The figure shows three views and two pictorial views of one solid part (mm, origin at its lowest corner). Answer the questions. Round coordinates to 2 decimals unless told otherwise and drop trailing zeros. Order: outer loops, then holes, each group sorted by start corner. A loop starts at its lowest first (then second) coordinate and runs counter-clockwise, first axis right, second up. Notation, with made-up numbers: (-26, 40) - (10, 40) arc R21 cw to (10, 60) - close; hole circle Ø8 at (-5.5, -5.5). An arc over 180 degrees is marked (long way). Use CSV: the item, a comma, the result in double quotes. Start each with the question number.
Item 1: Find section A-A, the plane y = 10. Give the vertices of the cut face in (x, z).
Item 2: Flat-ended cylindrical pins translate along their axes: P1, Ø1.5, axis at x = 8.5, z = 0.5, coming from the +Y side (1 decimal); P2, Ø1.5, axis at x = 22.5, z = 1, coming from the +Y side (1 decimal); P3, Ø1.7, axis at x = 43.25, y = 10, coming from the -Z side; P4, Ø1, axis at y = 44.5, z = 0.5, coming from the -X side. Find the tip coordinate at first contact, or state that the pin passes through.
Item 3: Find section B-B, the plane x = 9. Give the vertices of the cut face in (y, z) (1 decimal), plus the area to 3 significant figures.
Item 4: Find section C-C, the plane z = 2.35. Give the vertices of the cut face in (x, y), plus the area to 3 significant figures.
Item 5: Straight lines are drawn through the part: line 1 along X through (y, z) = (19, 0.45); line 2 along Y through (x, z) = (27.5, 0.65) (1 decimal); line 3 along Y through (x, z) = (45, 1.5) (1 decimal). For each, find the intervals that lie inside material, in ascending order. Write a range as [from, to].
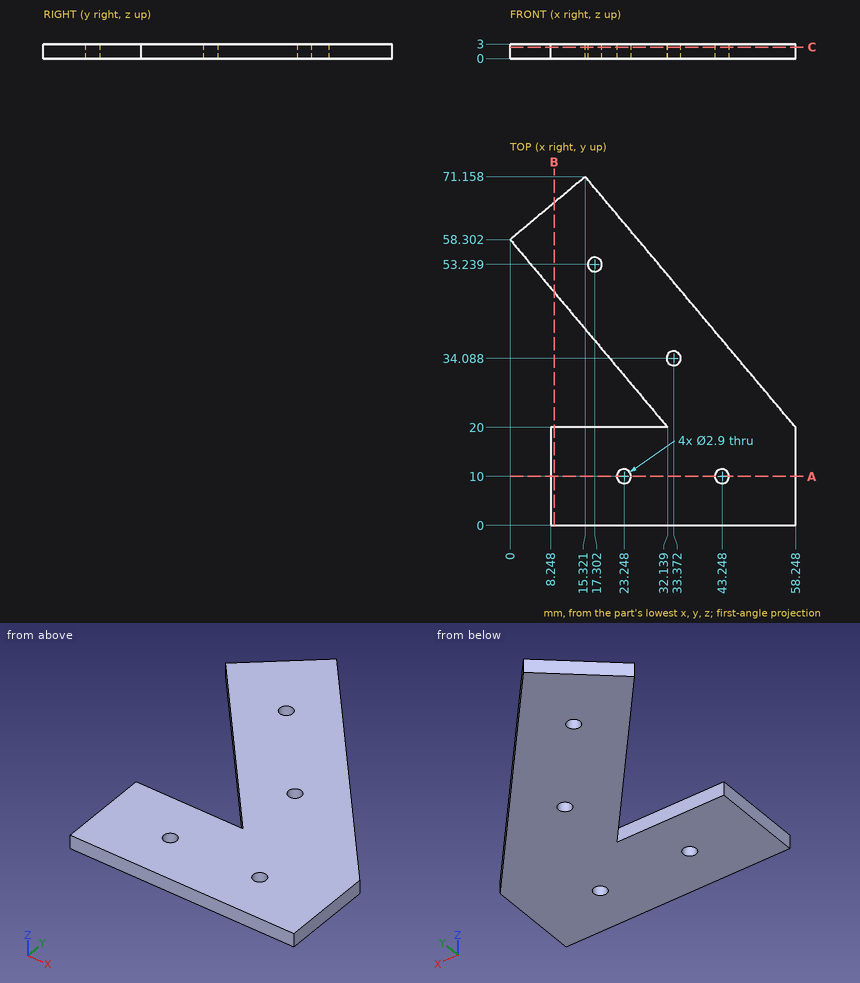
Worked out:
1,outline,"(8.25, 0) - (21.8, 0) - (21.8, 3) - (8.25, 3) - close; (24.7, 0) - (41.8, 0) - (41.8, 3) - (24.7, 3) - close; (44.7, 0) - (58.25, 0) - (58.25, 3) - (44.7, 3) - close"
2,P1,"stops at y = 66.1"
2,P2,"stops at y = 63.5"
2,P3,"passes through"
2,P4,"stops at x = 11.16"
3,outline,"(0, 0) - (20, 0) - (20, 3) - (0, 3) - close; (47.6, 0) - (65.9, 0) - (65.9, 3) - (47.6, 3) - close"
3,area,"115 mm²"
4,outline,"(0, 58.3) - (32.14, 20) - (8.25, 20) - (8.25, 0) - (58.25, 0) - (58.25, 20) - (15.32, 71.16) - close; hole circle Ø2.9 at (17.3, 53.24); hole circle Ø2.9 at (23.25, 10); hole circle Ø2.9 at (33.37, 34.09); hole circle Ø2.9 at (43.25, 10)"
4,area,"2,140 mm²"
5,line 1,"x = [8.25, 58.25]"
5,line 2,"y = [0, 20], [25.5, 56.6]"
5,line 3,"y = [0, 35.8]"
